Geometry check sheet. Reference: the model listing, model coordinates, mm. Coordinates: 2 decimals unless noted, no trailing zeros. Loops run counter-clockwise (first coordinate to the right, second up) from the corner with the lowest first, then second, coordinate; pieces in that order, holes last.
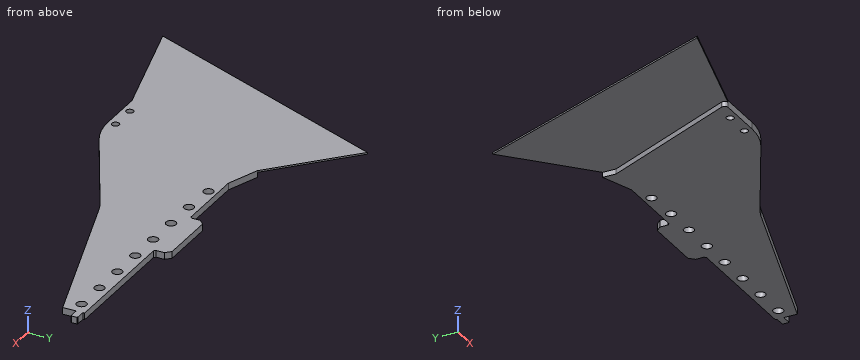
from build123d import *

# Parameters (mm, degrees)
SKETCH_1_R      = 1.1
SKETCH_1_R_2    = 1.5
EXTRUDE_1_DEPTH = 2
EXTRUDE_START   = -0.5
EXTRUDE_2_DEPTH = 0.5


with BuildPart() as part:
    # 草图1 → 凸台-拉伸1 (new body)
    with BuildSketch(Plane.XY):
        with BuildLine():
            Line((56.016004386, 19), (53.216004386, 19))
            Line((53.216004386, 19), (53.216004386, 19.5))
            Line((53.216004386, 19.5), (14.716004386, 19.5))
            Line((14.716004386, 19.5), (14.216004386, 20))
            Line((14.216004386, 20), (14.216004386, 22.5))
            Line((14.216004386, 22.5), (12.716004386, 24))
            Line((12.716004386, 24), (-4.283995614, 24))
            Line((-4.283995614, 24), (-5.783995614, 22.5))
            Line((-5.783995614, 22.5), (-5.783995614, 20))
            Line((-5.783995614, 20), (-6.283995614, 19.5))
            Line((-6.283995614, 19.5), (-27.158995614, 19.5))
            Line((-27.158995614, 19.5), (-36.783995614, 23))
            Line((-36.783995614, 23), (-36.783995614, 19))
            Line((-36.783995614, 19), (-56.122725498, -22.57826925))
            ThreePointArc((-56.122725498, -22.57826925), (-56.059132712, -23.5377124), (-55.216004386, -24))
            Line((-55.216004386, -24), (-41.838790186, -24))
            ThreePointArc((-41.838790186, -24), (-36.938094618, -23.390285788), (-32.336201424, -21.598318295))
            Line((-32.336201424, -21.598318295), (-1.744334209, -5.079584588))
            ThreePointArc((-1.744334209, -5.079584588), (-0.095831441, -4.284607006), (1.618440476, -3.643652619))
            Line((1.618440476, -3.643652619), (53.216004386, 13))
            Line((53.216004386, 13), (53.216004386, 17))
            Line((53.216004386, 17), (56.016004386, 17))
            Line((56.016004386, 17), (56.216004386, 17.2))
            Line((56.216004386, 17.2), (56.216004386, 18.8))
            Line((56.216004386, 18.8), (56.016004386, 19))
        make_face()
        with Locations((-41.838790186, -21.75)):
            Circle(SKETCH_1_R, mode=Mode.SUBTRACT)
        with Locations((-49.838790186, -21.75)):
            Circle(SKETCH_1_R, mode=Mode.SUBTRACT)
        with Locations((49.216004386, 16.5)):
            Circle(SKETCH_1_R_2, mode=Mode.SUBTRACT)
        with Locations((39.216004386, 16.5)):
            Circle(SKETCH_1_R_2, mode=Mode.SUBTRACT)
        with Locations((29.216004386, 16.5)):
            Circle(SKETCH_1_R_2, mode=Mode.SUBTRACT)
        with Locations((19.216004386, 16.5)):
            Circle(SKETCH_1_R_2, mode=Mode.SUBTRACT)
        with Locations((9.216004386, 16.5)):
            Circle(SKETCH_1_R_2, mode=Mode.SUBTRACT)
        with Locations((-0.783995614, 16.5)):
            Circle(SKETCH_1_R_2, mode=Mode.SUBTRACT)
        with Locations((-10.783995614, 16.5)):
            Circle(SKETCH_1_R_2, mode=Mode.SUBTRACT)
        with Locations((-20.783995614, 17)):
            Circle(SKETCH_1_R_2, mode=Mode.SUBTRACT)
    extrude(amount=EXTRUDE_1_DEPTH)

    # 草图2 → 凸台-拉伸2 (add)
    with BuildSketch(Plane.XY.offset(2).offset(EXTRUDE_START)):
        with BuildLine():
            Line((-55.216004386, -24), (-90.216004386, -33.41495792))
            Line((-90.216004386, -33.41495792), (-59.114143441, 43.782364027))
            Line((-59.114143441, 43.782364027), (-36.783995614, 23))
            Line((-36.783995614, 23), (-36.783995614, 19))
            Line((-36.783995614, 19), (-56.122725498, -22.57826925))
            ThreePointArc((-56.122725498, -22.57826925), (-56.059132712, -23.5377124), (-55.216004386, -24))
        make_face()
    extrude(amount=EXTRUDE_2_DEPTH)


solid = part.part
(1) Sectioned sample at C-C on x = -16. Record the cut outline in (y, z), and give its area (3 significant figures).
Findings:
outline: (-12.78, 0) - (19.5, 0) - (19.5, 2) - (-12.78, 2) - close
area: 64.6 mm2
(2) Sectioned sample at A-A on z = 0.9. State how many separate pieces and enclosed holes the cut face has, and give its area (3 significant figures).
Findings:
separate pieces: 1
enclosed holes: 10
area: 2,510 mm2
(3) Sectioned sample at B-B on y = 25.5. Record the cut outline in (x, z), and give its area (3 significant figures).
Findings:
outline: (-66.48, 1.5) - (-39.47, 1.5) - (-39.47, 2) - (-66.48, 2) - close
area: 13.5 mm2
(4) Gauge pin test, flat ends, axial feed: pin 1 Ø5 at (x, y) = (-55.5, 19) entering from -Z; pin 2 Ø1 at (y, z) = (21, 0.5) entering from -X. Record the tip position at first contact, or that the pin passes through.
Findings:
pin 1: stops at z = 1.5
pin 2: stops at x = -36.78
(5) Scan lines: L1, parallel to Y at x = 20.5, z = 1.1; L2, parallel to Z at x = -41, y = 20.5; L3, parallel to Y at x = 18.5, z = 0.25. Record each from-to range of solid material in increasing order.
Findings:
L1: y = 2.45 to 15.72, 17.28 to 19.5
L2: z = 1.5 to 2
L3: y = 1.8 to 15.18, 17.82 to 19.5
